from build123d import *

# Parameters (mm, degrees)
BOSS_EXTRUDE1_DEPTH = 6
BOSS_EXTRUDE2_DEPTH = 24.6
BOSS_EXTRUDE3_DEPTH = 6


with BuildPart() as part:
    # Sketch1 → Boss-Extrude1 (new body)
    with BuildSketch(Plane.XY):
        with BuildLine():
            Line((0, 0), (20, 0))
            Line((20, 0), (20, 4))
            Line((20, 4), (23.1, 4))
            Line((23.1, 4), (23.1, 11))
            Line((23.1, 11), (18, 11))
            ThreePointArc((18, 11), (10, 19), (2, 11))
            Line((2, 11), (-1.5, 11))
            Line((-1.5, 11), (-1.5, 4))
            Line((-1.5, 4), (0, 4))
            Line((0, 4), (0, 0))
        make_face()
        Polygon((13, 11), (11.5, 13.598076211), (8.5, 13.598076211), (7, 11), (8.5, 8.401923789), (11.5, 8.401923789), align=None, mode=Mode.SUBTRACT)
    extrude(amount=BOSS_EXTRUDE1_DEPTH)

    # Sketch2 → Boss-Extrude2 (add)
    with BuildSketch(Plane.ZY.offset(1.5)):
        with BuildLine():
            Line((6, 4), (6, 5))
            ThreePointArc((6, 5), (6.292893219, 4.292893219), (7, 4))
            Line((7, 4), (6, 4))
        make_face()
    extrude(amount=-BOSS_EXTRUDE2_DEPTH)

    # Sketch4 → Boss-Extrude3 (add)
    with BuildSketch(Plane.XY.offset(6)):
        with BuildLine():
            Line((23.1, 4), (23.1, 5))
            ThreePointArc((23.1, 5), (23.392893219, 4.292893219), (24.1, 4))
            Line((24.1, 4), (23.1, 4))
        make_face()
        with BuildLine():
            Line((-1.5, 4), (-2.5, 4))
            ThreePointArc((-2.5, 4), (-1.792893219, 4.292893219), (-1.5, 5))
            Line((-1.5, 5), (-1.5, 4))
        make_face()
    extrude(amount=-BOSS_EXTRUDE3_DEPTH)


solid = part.part
For this review, take the finished solid that the model builds, in its own axes (mm). A direction names the side the tool comes from. Coordinates: 2 decimals unless noted, no trailing zeros. Order: outer loops, then holes, each group sorted by start corner. A loop starts at its lowest first (then second) coordinate and runs counter-clockwise, first axis right, second up. Notation, with made-up numbers: (-18.5, 71.25) -> (19.5, 71.25) arc R32 cw to (19.5, 102.25) -> close; hole circle Ø5 at (-14, 5.25). An arc over 180 degrees is marked (long way). Return JSON: item names as keys, results as strings.
1. We need section B-B on z = 5.5. Write out the cut boundary in (x, y).
Answer block:
{"outline": "(-2.5, 4) -> (0, 4) -> (0, 0) -> (20, 0) -> (20, 4) -> (24.1, 4) arc R1 cw to (23.1, 5) -> (23.1, 11) -> (18, 11) arc R8 ccw to (2, 11) -> (-1.5, 11) -> (-1.5, 5) arc R1 cw to start; hole (7, 11) -> (8.5, 8.4) -> (11.5, 8.4) -> (13, 11) -> (11.5, 13.6) -> (8.5, 13.6) -> close"}
2. Machinability: for faces 1 (the flat face through (10, 2, 6)), 2 (the flat face through (23.1, 8, 3)), 3 (the flat face through (13.4, 10.5, 6)), 4 (the flat face through (7.76, 12.32, 2.96)), which of the approach directions +Z, -Z, +X, -X, +Y, -Y give a long, thin tool a straight path to every point of the face, cutting with its end or side? Answer none if there is none.
Answer block:
{"face 1": "+Z, +X, -X, -Y", "face 2": "+Z, -Z, +X, +Y", "face 3": "+Z, +X, -X, +Y", "face 4": "+Z, -Z"}
3. For line 1 (Y direction, x = 20.25, z = 4.25); line 2 (Y direction, x = 0.25, z = 4.25); line 3 (Z direction, x = 11.75, y = 2.5), list the stretches that pass through material, from the lowest coordinate up. Write a range as from..to.
Answer block:
{"line 1": "4..11", "line 2": "0..11", "line 3": "0..6"}
4. The part is to be moulded in two halves that separate along X. For faces 5 (the flat face through (12.26, 12.28, 2.96)), 6 (the flat face through (12.8, 4, 6.4)), 7 (the cylindrical face through (10, 19, 3)), say which applies: +X half, -X half, draft (parallel to the pull), parting line (faces both ways), or undercut.
Answer block:
{"face 5": "undercut", "face 6": "draft", "face 7": "parting line"}
5. We need section C-C on y = 13. Write out the cut boundary in (x, z).
Answer block:
{"outline": "(2.25, 0) -> (8.15, 0) -> (8.15, 6) -> (2.25, 6) -> close; (11.85, 0) -> (17.75, 0) -> (17.75, 6) -> (11.85, 6) -> close"}
6. We need section A-A on x = 10. Write out the cut boundary in (y, z), and give its area (3 significant figures).
Answer block:
{"outline": "(0, 0) -> (8.4, 0) -> (8.4, 6) -> (5, 6) arc R1 cw to (4, 7) -> (4, 6) -> (0, 6) -> close; (13.6, 0) -> (19, 0) -> (19, 6) -> (13.6, 6) -> close", "area": "83.0 mm²"}
7. We need section D-D on x = 13.5. Write out the cut boundary in (y, z).
Answer block:
{"outline": "(0, 0) -> (18.19, 0) -> (18.19, 6) -> (5, 6) arc R1 cw to (4, 7) -> (4, 6) -> (0, 6) -> close"}
8. For pin 1 Ø1.2 at (y, z) = (2, 3) entering from +X; pin 2 Ø2 at (y, z) = (2.5, 4) entering from -X; pin 3 Ø1.5 at (x, y) = (16.5, 11.5) entering from +Z, all flat-tipped, find the tip position at first contact; note any pin that passes through.
Answer block:
{"pin 1": "x = 20", "pin 2": "x = 0", "pin 3": "z = 6"}
